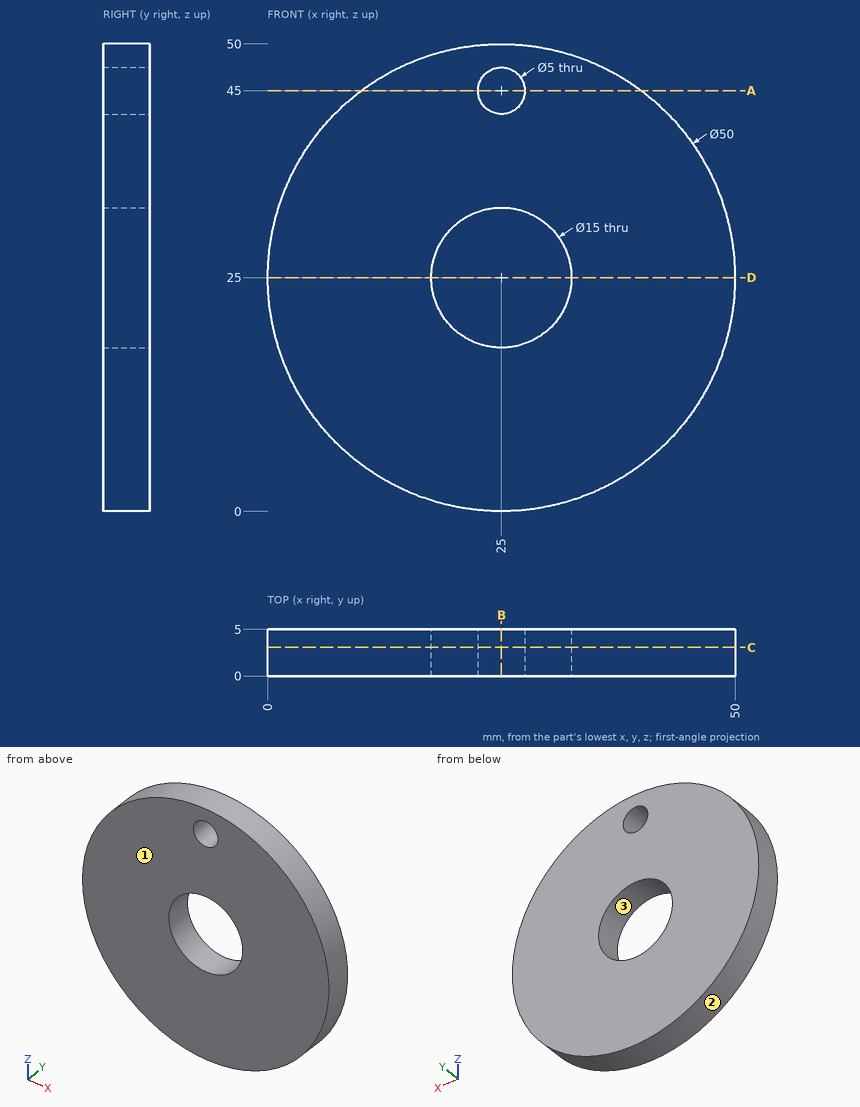
Answer from the drawing. Dimensions are ordinates in mm from the lowest x, y and z of the part. Coordinates: 2 decimals unless noted, no trailing zeros. Loops run counter-clockwise (first coordinate to the right, second up) from the corner with the lowest first, then second, coordinate; pieces in that order, holes last.
1) Section A-A (z = 45) is taken. Give the vertices of the cut face in (x, y).
Results:
outline: (10, 0) - (22.5, 0) - (22.5, 5) - (10, 5) - close; (27.5, 0) - (40, 0) - (40, 5) - (27.5, 5) - close
2) Flat-ended cylindrical pins translate along their axes: pin 1 (4.5 mm diameter, centred on x = 25, z = 45, fed in from -Y); pin 2 (1.5 mm diameter, centred on x = 23, y = 1.5, fed in from -Z); pin 3 (3 mm diameter, centred on x = 30, y = 4.5, fed in from -Z). Find the tip coordinate at first contact, or state that the pin passes through.
Results:
pin 1: passes through
pin 2: stops at z = 0.03
pin 3: stops at z = 0.25
3) Consider probe 1 along Z at (x, y) = (25, 1.8); probe 2 along X at (y, z) = (3.6, 45); probe 3 along X at (y, z) = (1.25, 30). Determine where each line is inside the solid, lowest interval first.
Results:
probe 1: z = 0 to 17.5, 32.5 to 42.5, 47.5 to 50
probe 2: x = 10 to 22.5, 27.5 to 40
probe 3: x = 0.51 to 19.41, 30.59 to 49.49
4) For a pull along X with two mould halves and no side action, classify the marked faces 1, 2 and 3 as +X half, -X half, draft (parallel to the pull), parting line (faces both ways), or undercut.
Results:
face 1: draft
face 2: parting line
face 3: undercut
5) Section D-D (z = 25) is taken. Give the vertices of the cut face in (x, y), plus the area to 3 significant figures.
Results:
outline: (0, 0) - (17.5, 0) - (17.5, 5) - (0, 5) - close; (32.5, 0) - (50, 0) - (50, 5) - (32.5, 5) - close
area: 175 mm2
6) Section B-B (x = 25) is taken. Give the vertices of the cut face in (y, z), plus the area to 3 significant figures.
Results:
outline: (0, 0) - (5, 0) - (5, 17.5) - (0, 17.5) - close; (0, 32.5) - (5, 32.5) - (5, 42.5) - (0, 42.5) - close; (0, 47.5) - (5, 47.5) - (5, 50) - (0, 50) - close
area: 150 mm2
7) Section C-C (y = 3.05) is taken. Give the vertices of the cut face in (x, z).
Results:
outline: circle Ø50 at (25, 25); hole circle Ø15 at (25, 25); hole circle Ø5 at (25, 45)
